```python
from build123d import *

# Parameters (mm, degrees)
BOSS_EXTRU_1_DEPTH = 24


with BuildPart() as part:
    # Esquisse1 → Boss.-Extru.1 (new body)
    with BuildSketch(Plane(origin=(0, 0, 0), x_dir=(0, 0, -1), z_dir=(1, 0, 0))):
        Polygon((-9.5, -5.484827557), (-9.5, 5.484827557), (0, 10.969655115), (9.5, 5.484827557), (9.5, -5.484827557), (0, -10.969655115), align=None)
        with BuildLine():
            Line((2.25, 6.25), (-2.25, 6.25))
            ThreePointArc((-2.25, 6.25), (-4.017766953, 5.517766953), (-4.75, 3.75))
            Line((-4.75, 3.75), (-4.75, -3.75))
            ThreePointArc((-4.75, -3.75), (-4.017766953, -5.517766953), (-2.25, -6.25))
            Line((-2.25, -6.25), (2.25, -6.25))
            ThreePointArc((2.25, -6.25), (4.017766953, -5.517766953), (4.75, -3.75))
            Line((4.75, -3.75), (4.75, 3.75))
            ThreePointArc((4.75, 3.75), (4.017766953, 5.517766953), (2.25, 6.25))
        make_face(mode=Mode.SUBTRACT)
    extrude(amount=BOSS_EXTRU_1_DEPTH)

    # Esquisse6 → Enlèvement de matière-Révolution1 (revolve, cut)
    with BuildSketch(Plane(origin=(0, 0, 0), x_dir=(1, 0, 0), z_dir=(0, 1, 0))):
        Polygon((-4.48433242, 1.732908411), (2.760156758, 14.280731742), (21.239843242, 14.280731742), (28.008759285, 2.556625243), (28.008759285, 15.540866197), (-4.48433242, 15.540866197), align=None)
    revolve(axis=Axis((24, 0, 0), (-1, 0, 0)), mode=Mode.SUBTRACT)

    # Esquisse11 → Enlèvement de matière-Révolution3 (revolve, cut)
    with BuildSketch(Plane(origin=(0, 0, 0), x_dir=(1, 0, 0), z_dir=(0, 1, 0)), mode=Mode.PRIVATE) as enl_vement_de_mati_re_r_volution3_sk:
        Polygon((0, 0), (0, -7), (3, -4), (21, -4), (24, -7), (24, 0), align=None)
    revolve(enl_vement_de_mati_re_r_volution3_sk.sketch.rotate(Axis((24, 0, 0), (-1, 0, 0)), 180), axis=Axis((24, 0, 0), (-1, 0, 0)), mode=Mode.SUBTRACT)  # turned: the seam where the file's is


solid = part.part
```
Model file for the job. Use its own axes, mm. A direction names the side the tool comes from. Give positions to 0.01 mm unless a question says otherwise; leave off trailing zeros. Order: outer loops, then holes, each group sorted by start corner. A loop starts at its lowest first (then second) coordinate and runs counter-clockwise, first axis right, second up.
1) Saw through at A-A, the plane x = 5. Write the cut outline in (y, z), then the cut area to 3 significant figures.
2) 3-axis set-ups, long thin cutter, end or side, ignore diameter. For faces 1 (the conical face through (0.21, -9.86, -0.02)), 2 (the flat face through (12, 6.25, 0)): which of +Z, -Z, +X, -X, +Y, -Y reach the whole face in a straight line?
3) Pin check, flat tips, straight feed: pin 1 (1 mm diameter, centred on x = 13, z = 2, fed in from -Y); pin 2 (1.5 mm diameter, centred on x = 21.5, z = 3.5, fed in from -Y); pin 3 (1 mm diameter, centred on x = 2.5, y = 7, fed in from +Z). Stop position of each tip, or through.
4) Wall check: probe 1 along Z at (x, y) = (5, -3); probe 2 along Z at (x, y) = (12.75, -5.75); probe 3 along Y at (x, z) = (5.5, 2.5). Give the ranges that are in metal, low to high.
5) Saw through at B-B, the plane x = 22.25. Write the cut outline in (y, z).
6) Mould opens along Z. For faces 3 (the conical face through (23.8, -9.85, -0.02)), 4 (the flat face through (12, -6.25, 0)), 5 (the conical face through (0.206, 4.949, -8.525)) say: +Z half, -Z half, draft (parallel to the pull), parting line (faces both ways), or undercut.
Computed:
1. outline: (-10.97, 0) - (-5.48, -9.5) - (5.48, -9.5) - (10.97, 0) - (5.48, 9.5) - (-5.48, 9.5) - close; hole (-6.25, -2.25) arc R2.5 ccw to (-3.75, -4.75) - (3.75, -4.75) arc R2.5 ccw to (6.25, -2.25) - (6.25, 2.25) arc R2.5 ccw to (3.75, 4.75) - (-3.75, 4.75) arc R2.5 ccw to (-6.25, 2.25) - close
1. area: 199 mm2
2. face 1: -X, -Y
2. face 2: +X, -X
3. pin 1: stops at y = -10.1
3. pin 2: stops at y = -9.38
3. pin 3: stops at z = 7.74
4. probe 1: z = -9.5 to -4.75, 4.75 to 9.5
4. probe 2: z = -9.04 to -3.75, 3.75 to 9.04
4. probe 3: y = -9.53 to -6.24, 6.24 to 9.53
5. outline: (-10.97, 0) - (-5.48, -9.5) - (5.48, -9.5) - (10.97, 0) - (5.48, 9.5) - (-5.48, 9.5) - close; hole (-6.25, -2.25) arc R2.5 ccw to (-3.75, -4.75) - (-2.24, -4.75) arc R5.25 ccw to (2.24, -4.75) - (3.75, -4.75) arc R2.5 ccw to (6.25, -2.25) - (6.25, 2.25) arc R2.5 ccw to (3.75, 4.75) - (2.24, 4.75) arc R5.25 ccw to (-2.24, 4.75) - (-3.75, 4.75) arc R2.5 ccw to (-6.25, 2.25) - close
6. face 3: parting line
6. face 4: undercut
6. face 5: -Z half
